Model file for the job. Use its own axes, mm. A direction names the side the tool comes from. Coordinates: 2 decimals unless noted, no trailing zeros. Loops run counter-clockwise (first coordinate to the right, second up) from the corner with the lowest first, then second, coordinate; pieces in that order, holes last. Notation, with made-up numbers: (62, 66.5) -> (121, 66.5) arc R30 cw to (121, 98.5) -> close; hole circle Ø5 at (28, 58.5). An arc over 180 degrees is marked (long way). Use one line per item in the form item = value.
```python
from build123d import *

# Parameters (mm, degrees)
SKETCH1_W           = 20
SKETCH1_H           = 10
BOSS_EXTRUDE1_DEPTH = 38.5
SKETCH5_W           = 16
SKETCH5_H           = 30.5
BOSS_EXTRUDE2_DEPTH = 8
SKETCH2_R           = 5.1
CUT_EXTRUDE3_DEPTH  = 10
FILLET1_R           = 2
SKETCH6_W           = 23.5
SKETCH6_H           = 20
CUT_EXTRUDE4_DEPTH  = 8
SKETCH7_W           = 2.2
SKETCH7_H           = 2.2
CUT_EXTRUDE5_DEPTH  = 3
SKETCH8_W           = 30.5
SKETCH8_H           = 2
BOSS_EXTRUDE3_DEPTH = 2


with BuildPart() as part:
    # Sketch1 → Boss-Extrude1 (new body)
    with BuildSketch(Plane.YZ):
        Rectangle(SKETCH1_W, SKETCH1_H)
    extrude(amount=BOSS_EXTRUDE1_DEPTH)

    # Sketch5 → Boss-Extrude2 (add)
    with BuildSketch(Plane(origin=(0, 0, 0), x_dir=(0, 1, 0), z_dir=(0, 0, 1))):
        with Locations((0, -21.25)):
            Rectangle(SKETCH5_W, SKETCH5_H)
    extrude(amount=BOSS_EXTRUDE2_DEPTH)

    # Sketch2 → Cut-Extrude3 (cut)
    with BuildSketch(Plane.YZ):
        Circle(SKETCH2_R)
    extrude(amount=CUT_EXTRUDE3_DEPTH, mode=Mode.SUBTRACT)

    # Fillet1
    fillet1_edges = [part.edges().sort_by_distance(p)[0] for p in [
        (19.25, 10, -5),
        (19.25, -10, -5),
    ]]
    fillet(fillet1_edges, radius=FILLET1_R)

    # Sketch6 → Cut-Extrude4 (cut)
    with BuildSketch(Plane(origin=(0, 0, -5), x_dir=(1, 0, 0), z_dir=(0, 0, -1))):
        with Locations((26.75, 0)):
            Rectangle(SKETCH6_W, SKETCH6_H)
    extrude(amount=-CUT_EXTRUDE4_DEPTH, mode=Mode.SUBTRACT)

    # Sketch7 → Cut-Extrude5 (cut)
    with BuildSketch(Plane.YZ.offset(15)):
        with Locations((6, 0)):
            Rectangle(SKETCH7_W, SKETCH7_H)
        with Locations((-6, 0)):
            Rectangle(SKETCH7_W, SKETCH7_H)
    extrude(amount=-CUT_EXTRUDE5_DEPTH, mode=Mode.SUBTRACT)

    # Sketch8 → Boss-Extrude3 (add)
    with BuildSketch(Plane.XY.offset(8)):
        with Locations((21.25, 7)):
            Rectangle(SKETCH8_W, SKETCH8_H)
        with Locations((21.25, -7)):
            Rectangle(SKETCH8_W, SKETCH8_H)
    extrude(amount=BOSS_EXTRUDE3_DEPTH)


solid = part.part
```
Q1. Band-saw the part on A-A, the plane y = 0. Write the cut outline in (x, z).
Result:
outline = (6, 5.1) -> (10, 5.1) -> (10, -5) -> (15, -5) -> (15, 3) -> (38.5, 3) -> (38.5, 5) -> (36.5, 5) -> (36.5, 8) -> (6, 8) -> close
Q2. Wall check: line 1 along Y through (x, z) = (6.75, 0); line 2 along X through (y, z) = (2.25, 2.5); line 3 along X through (y, z) = (6.5, -3.5). Give the ranges that are in metal, low to high.
Result:
line_1 = -10 to -5.1, 5.1 to 10
line_2 = 10 to 15
line_3 = 0 to 15
Q3. Which spindle directions (+Z, -Z, +X, -X, +Y, -Y) get a long thin tool onto all of the face, cutting with end or side? Do faces 1 (the face through (27, 0, 3)), 2 (the face through (14, 6, -1.1)), 3 (the face through (10, 0, 0)), 4 (the face through (21, 6, 9)). Say none if no direction does.
Result:
face_1 = -Z, +X, +Y, -Y
face_2 = +X
face_3 = -X
face_4 = +Z, +X, -X
Q4. Mould opens along Y. For faces 5 (the face through (7.6, -9.43, -4.4)), 6 (the face through (14, -6, 1.1)), 7 (the face through (6, 0, 7)) say: released by +Y, released by -Y, zero draft, split by the parting line, or undercut.
Result:
face_5 = released by -Y
face_6 = undercut
face_7 = zero draft
Q5. Band-saw the part on C-C, the plane z = 0. Write the cut outline in (x, y), and give its area (3 significant figures).
Result:
outline = (0, -10) -> (15, -10) -> (15, -7.1) -> (12, -7.1) -> (12, -4.9) -> (15, -4.9) -> (15, 4.9) -> (12, 4.9) -> (12, 7.1) -> (15, 7.1) -> (15, 10) -> (0, 10) -> (0, 5.1) -> (10, 5.1) -> (10, -5.1) -> (0, -5.1) -> close
area = 185 mm2
Q6. Band-saw the part on B-B, the plane x = 14. Write the cut outline in (y, z), and give its area (3 significant figures).
Result:
outline = (-10, -3) arc R2 ccw to (-8, -5) -> (8, -5) arc R2 ccw to (10, -3) -> (10, 5) -> (8, 5) -> (8, 10) -> (6, 10) -> (6, 8) -> (-6, 8) -> (-6, 10) -> (-8, 10) -> (-8, 5) -> (-10, 5) -> close; hole (-7.1, -1.1) -> (-4.9, -1.1) -> (-4.9, 1.1) -> (-7.1, 1.1) -> close; hole (4.9, -1.1) -> (7.1, -1.1) -> (7.1, 1.1) -> (4.9, 1.1) -> close
area = 245 mm2
Q7. Pin check, flat tips, straight feed: pin 1 Ø1 at (x, y) = (24.5, -4) entering from +Z; pin 2 Ø0.6 at (x, z) = (24, 8.5) entering from -Y; pin 3 Ø3 at (x, z) = (17, -1) entering from -Y; pin 4 Ø1.8 at (y, z) = (6.5, 0) entering from +X. Stop position of each tip, or through.
Result:
pin_1 = 8
pin_2 = -8
pin_3 = through
pin_4 = 15
Q8. Band-saw the part on D-D, the plane x = 34.5. Write the cut outline in (y, z).
Result:
outline = (-10, 3) -> (10, 3) -> (10, 5) -> (8, 5) -> (8, 10) -> (6, 10) -> (6, 8) -> (-6, 8) -> (-6, 10) -> (-8, 10) -> (-8, 5) -> (-10, 5) -> close
